Check sheet for the modelled part. Datum: model origin and axes. Units: mm. Give positions to 0.01 mm unless a question says otherwise; leave off trailing zeros. Loops run counter-clockwise (first coordinate to the right, second up) from the corner with the lowest first, then second, coordinate; pieces in that order, holes last. Notation, with made-up numbers: (2, 32) -> (60, 32) arc R26 cw to (60, 58) -> close; hole circle Ø6 at (-14.75, 53.5). An arc over 180 degrees is marked (long way). Write each question's results on one line, items separated by ' | '. Start each with the question number.
Item 1: Cross-section at A-A on y = -100. Enter the section's corners in (x, z), then the cut area to 3 significant figures.
Item 2: Cross-section at B-B on x = -175. State how many separate pieces and enclosed holes the cut face has, then the cut area to 3 significant figures.
Item 3: Scan lines: line 1 along Y through (x, z) = (-75, 1.5); line 2 along Y through (x, z) = (-74, 0.6); line 3 along X through (y, z) = (-103, 0.4). Record each from-to range of solid material in increasing order.
Item 4: Cross-section at C-C on x = 25. Enter the section's corners in (y, z).
Item 5: Gauge pin test, flat ends, axial feed: pin 1 Ø13 at (x, y) = (-25, 150) entering from +Z; pin 2 Ø21 at (x, y) = (175, -100) entering from -Z. Record the tip position at first contact, or that the pin passes through.
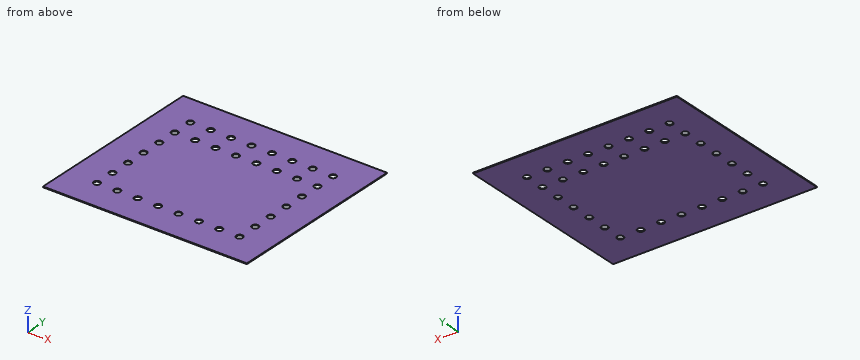
from build123d import *

# Parameters (mm, degrees)
F0_W     = 500
F0_H     = 450
F0_R     = 8
F1_DEPTH = 2


with BuildPart() as f1:
    # F0 (on Top) → F1 (new body)
    with BuildSketch(Plane.XY):
        Rectangle(F0_W, F0_H)
        with Locations((-175, -150)):
            Circle(F0_R, mode=Mode.SUBTRACT)
        with Locations((-125, -150)):
            Circle(F0_R, mode=Mode.SUBTRACT)
        with Locations((-75, -150)):
            Circle(F0_R, mode=Mode.SUBTRACT)
        with Locations((-25, -150)):
            Circle(F0_R, mode=Mode.SUBTRACT)
        with Locations((-175, -100)):
            Circle(F0_R, mode=Mode.SUBTRACT)
        with Locations((-175, -50)):
            Circle(F0_R, mode=Mode.SUBTRACT)
        with Locations((25, -150)):
            Circle(F0_R, mode=Mode.SUBTRACT)
        with Locations((75, -150)):
            Circle(F0_R, mode=Mode.SUBTRACT)
        with Locations((125, -150)):
            Circle(F0_R, mode=Mode.SUBTRACT)
        with Locations((175, -150)):
            Circle(F0_R, mode=Mode.SUBTRACT)
        with Locations((175, -100)):
            Circle(F0_R, mode=Mode.SUBTRACT)
        with Locations((175, -50)):
            Circle(F0_R, mode=Mode.SUBTRACT)
        with Locations((-175, 0)):
            Circle(F0_R, mode=Mode.SUBTRACT)
        with Locations((-175, 50)):
            Circle(F0_R, mode=Mode.SUBTRACT)
        with Locations((-175, 100)):
            Circle(F0_R, mode=Mode.SUBTRACT)
        with Locations((-125, 100)):
            Circle(F0_R, mode=Mode.SUBTRACT)
        with Locations((-75, 100)):
            Circle(F0_R, mode=Mode.SUBTRACT)
        with Locations((-25, 100)):
            Circle(F0_R, mode=Mode.SUBTRACT)
        with Locations((-175, 150)):
            Circle(F0_R, mode=Mode.SUBTRACT)
        with Locations((-125, 150)):
            Circle(F0_R, mode=Mode.SUBTRACT)
        with Locations((-75, 150)):
            Circle(F0_R, mode=Mode.SUBTRACT)
        with Locations((-25, 150)):
            Circle(F0_R, mode=Mode.SUBTRACT)
        with Locations((25, 100)):
            Circle(F0_R, mode=Mode.SUBTRACT)
        with Locations((75, 100)):
            Circle(F0_R, mode=Mode.SUBTRACT)
        with Locations((175, 0)):
            Circle(F0_R, mode=Mode.SUBTRACT)
        with Locations((175, 50)):
            Circle(F0_R, mode=Mode.SUBTRACT)
        with Locations((125, 100)):
            Circle(F0_R, mode=Mode.SUBTRACT)
        with Locations((175, 100)):
            Circle(F0_R, mode=Mode.SUBTRACT)
        with Locations((25, 150)):
            Circle(F0_R, mode=Mode.SUBTRACT)
        with Locations((75, 150)):
            Circle(F0_R, mode=Mode.SUBTRACT)
        with Locations((125, 150)):
            Circle(F0_R, mode=Mode.SUBTRACT)
        with Locations((175, 150)):
            Circle(F0_R, mode=Mode.SUBTRACT)
    extrude(amount=F1_DEPTH)


solid = f1.part
Answer sheet:
1) outline: (-250, 0) -> (-183, 0) -> (-183, 2) -> (-250, 2) -> close; (-167, 0) -> (167, 0) -> (167, 2) -> (-167, 2) -> close; (183, 0) -> (250, 0) -> (250, 2) -> (183, 2) -> close | area: 936 mm²
2) separate pieces: 8 | enclosed holes: 0 | area: 676 mm²
3) line 1: y = -225 to -158, -142 to 92, 108 to 142, 158 to 225 | line 2: y = -225 to -157.94, -142.06 to 92.06, 107.94 to 142.06, 157.94 to 225 | line 3: x = -250 to -182.42, -167.58 to 167.58, 182.42 to 250
4) outline: (-225, 0) -> (-158, 0) -> (-158, 2) -> (-225, 2) -> close; (-142, 0) -> (92, 0) -> (92, 2) -> (-142, 2) -> close; (108, 0) -> (142, 0) -> (142, 2) -> (108, 2) -> close; (158, 0) -> (225, 0) -> (225, 2) -> (158, 2) -> close
5) pin 1: passes through | pin 2: stops at z = 0
